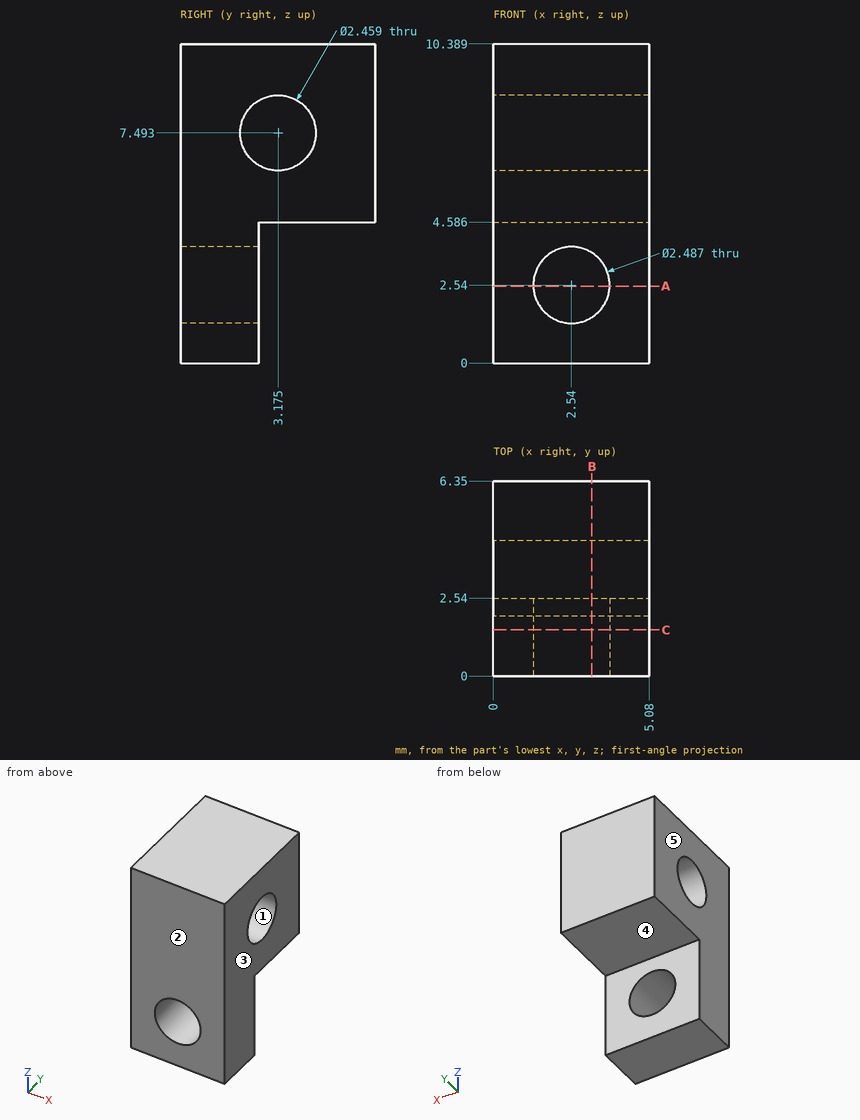
Can you work these out from the drawing? Everything is in mm from the part's minimum corner. A direction names the side the tool comes from. Coordinates: 2 decimals unless noted, no trailing zeros. Write each loop counter-clockwise with the first axis right and the second up, starting at its lowest first coordinate (ties: lowest second). Pieces come first, ordered by that corner, then holes. Notation, with made-up numbers: (4.25, 50.25) -> (51.25, 50.25) arc R21 cw to (51.25, 70.25) -> close; hole circle Ø7 at (-18, -0.75). An arc over 180 degrees is marked (long way). Return JSON: item names as keys, results as strings.
(1) We'd pull the mould along Y, two halves only. Please class the marked faces 1, 2 and 3: +Y half, -Y half, draft (parallel to the pull), parting line (faces both ways), or undercut.
Numbers:
{"face 1": "undercut", "face 2": "-Y half", "face 3": "draft"}
(2) Which directions (+Z, -Z, +X, -X, +Y, -Y) give clear straight access to the entire face, cutting with the end or side of a thin tool? Please do the marked faces 4 and 5.
Numbers:
{"face 4": "-Z, +X, -X, +Y", "face 5": "+Z, -Z, -X, +Y, -Y"}
(3) Imagine slicing it at A-A, the plane z = 2.5. Please give me the cut outline in (x, y).
Numbers:
{"outline": "(0, 0) -> (1.3, 0) -> (1.3, 2.54) -> (0, 2.54) -> close; (3.78, 0) -> (5.08, 0) -> (5.08, 2.54) -> (3.78, 2.54) -> close"}
(4) Imagine slicing it at B-B, the plane x = 3.2. Count the separate pieces of the cut face and the enclosed holes in it, then the cut area to 3 significant figures.
Numbers:
{"separate pieces": "2", "enclosed holes": "1", "area": "38.4 mm2"}
(5) Imagine slicing it at C-C, the plane y = 1.5. Please give me the cut outline in (x, z).
Numbers:
{"outline": "(0, 0) -> (5.08, 0) -> (5.08, 10.39) -> (0, 10.39) -> close; hole circle Ø2.49 at (2.54, 2.54)"}
(6) I need wall thicknesses on L1, parallel to Z at x = 2.54, y = 1.1; L2, parallel to X at y = 2.5, z = 2.5; L3, parallel to Z at x = 3.3, y = 5.25. Which ranges of each line are inside material? Lowest first, please.
Numbers:
{"L1": "z = 0 to 1.3, 3.78 to 10.39", "L2": "x = 0 to 1.3, 3.78 to 5.08", "L3": "z = 4.59 to 10.39"}
(7) I'm going to push a flat-ended pin straight in: pin 1 (3 mm diameter, centred on x = 2.54, z = 2.54, fed in from +Y). Where does the tip first touch, or does it pass through?
Numbers:
{"pin 1": "stops at y = 2.54"}
